Can you work these out from the model? Positions are in its coordinate system, mm. A direction names the side the tool comes from. Give positions to 0.01 mm unless a question says otherwise; leave off trailing zeros. Loops run counter-clockwise (first coordinate to the right, second up) from the corner with the lowest first, then second, coordinate; pieces in that order, holes last. Notation, with made-up numbers: (49.5, -28.5) - (91.5, -28.5) arc R25 cw to (91.5, -10.5) - close; hole circle Ø9 at (-37, 86). An arc over 180 degrees is marked (long way). Answer as a JSON object with one key per item and string values. Group by question number.
Item 1: Which directions (+Z, -Z, +X, -X, +Y, -Y) give clear straight access to the entire face, cutting with the end or side of a thin tool? Please do faces 5 (the cylindrical face through (-0.314, -14.284, 3.863)), 6 (the cylindrical face through (6.983, 43.545, 3.863)), 7 (the flat face through (-9, 51.243, 4)).
Item 2: Suppose I cut it at B-B on y = 52.07. Write out the boundary of the cut face in (x, z), and give its area (3 significant figures).
Item 3: Please list where these lines run through material, in increasing order: L1, parallel to X at y = 52.5, z = 7.25; L2, parallel to Y at x = -7, z = 2.5; L3, parallel to X at y = 17.5, z = 1.25.
Item 4: Suppose I cut it at C-C on z = 1.5. Count the separate pieces of the cut face and the enclosed holes in it, and give its area (3 significant figures).
Item 5: Thinking about a two-plate mould opening in X: for faces 1 (the cylindrical face through (-11.94, 52.05, 3.86)), 2 (the flat face through (-3, 44.45, 4)), 3 (the flat face through (14.288, 27, 4)), 4 (the cylindrical face through (0.175, -7.936, 3.863)), which applies, pulls with the +X half, pulls with the -X half, needs draft (parallel to the pull), parting line crosses it, or undercut?
Item 6: Suppose I cut it at D-D on y = 2. Write out the boundary of the cut face in (x, z).
Item 7: Will these pins go through, and if not, where does the flat tip stop? pin 1 (2.5 mm diameter, centred on x = -2.5, z = 2.5, fed in from -Y); pin 2 (2.5 mm diameter, centred on y = 11.5, z = 2.5, fed in from -X); pin 3 (4 mm diameter, centred on x = -8, z = 3.5, fed in from +Y).
from build123d import *

# Parameters (mm, degrees)
F1_DEPTH = 3.81
F2_R     = 22.225
F3_DEPTH = 109
F4_DEPTH = 28.576


# Not quite as in the source:
# - an extrude ends at something that could not be found from the text; its depth is read off the source's solid
# - a pattern or mirror of a feature is missing from the dataset's text; its kind, count and spacing are read off the source's solid


with BuildPart() as f1:
    # F0 (on Top) → F1 (new body)
    with BuildSketch(Plane.XY):
        with BuildLine():
            ThreePointArc((7.9375, 0), (0, -7.9375), (-7.9375, 0))
            ThreePointArc((-7.9375, 0), (-8.8674359697, 2.2450640303), (-11.1125, 3.175))
            ThreePointArc((-11.1125, 3.175), (-13.3575640303, 2.2450640303), (-14.2875, 0))
            ThreePointArc((-14.2875, 0), (0, -14.2875), (14.2875, 0))
            Line((14.2875, 0), (14.2875, 53.975))
            ThreePointArc((14.2875, 53.975), (13.3575640303, 56.2200640303), (11.1125, 57.15))
            Line((11.1125, 57.15), (-11.1125, 57.15))
            ThreePointArc((-11.1125, 57.15), (-13.3575640303, 56.2200640303), (-14.2875, 53.975))
            Line((-14.2875, 53.975), (-14.2875, 47.625))
            ThreePointArc((-14.2875, 47.625), (-13.3575640303, 45.3799359697), (-11.1125, 44.45))
            Line((-11.1125, 44.45), (4.7625, 44.45))
            ThreePointArc((4.7625, 44.45), (7.0075640303, 43.5200640303), (7.9375, 41.275))
            Line((7.9375, 41.275), (7.9375, 0))
        make_face()
        with BuildLine():
            ThreePointArc((-11.1125, 51.2426083993), (-11.9398916007, 52.07), (-11.1125, 52.8973916007))
            Line((-11.1125, 52.8973916007), (-6.3490160938, 52.8936081389))
            ThreePointArc((-6.3490160938, 52.8936081389), (-5.5241718233, 52.0677805671), (-6.3496717582, 51.2426083993))
            Line((-6.3496717582, 51.2426083993), (-11.1125, 51.2426083993))
        make_face(mode=Mode.SUBTRACT)
        with BuildLine():
            ThreePointArc((11.1133453348, 52.8905930346), (11.93309347, 52.07), (11.1133453348, 51.2494069654))
            Line((11.1133453348, 51.2494069654), (6.35, 51.2445))
            ThreePointArc((6.35, 51.2445), (5.5245, 52.07), (6.35, 52.8955))
            Line((6.35, 52.8955), (11.1133453348, 52.8905930346))
        make_face(mode=Mode.SUBTRACT)
    extrude(amount=F1_DEPTH)

    # F1_copies: F1 across plane


with BuildPart() as f1_1:
    add(f1.part)
    add(f1.part.mirror(Plane.XY.offset(3.81)))

    # F2 (on face) → F3 (cut, through all)
    with BuildSketch(Plane(origin=(-14.2875, 0, 0), x_dir=(0, -1, 0), z_dir=(-1, 0, 0))):
        with Locations((79.121, 3.81)):
            Circle(F2_R)
        with BuildLine():
            ThreePointArc((-57.15, 0.4595098866), (-56.9595909744, 2.1299479175), (-56.896, 3.81))
            ThreePointArc((-56.896, 3.81), (-101.2824090256, 5.4900520825), (-57.15, 0.4595098866))
        make_face()
    extrude(amount=F3_DEPTH, mode=Mode.SUBTRACT)

    # F2 (on face) → F4 (cut, through all)
    with BuildSketch(Plane(origin=(-14.2875, 0, 0), x_dir=(0, -1, 0), z_dir=(-1, 0, 0))):
        with Locations((79.121, 3.81)):
            Circle(F2_R)
        with BuildLine():
            ThreePointArc((-57.15, 0.4595098866), (-56.9595909744, 2.1299479175), (-56.896, 3.81))
            ThreePointArc((-56.896, 3.81), (-101.2824090256, 5.4900520825), (-57.15, 0.4595098866))
        make_face()
    extrude(amount=-F4_DEPTH, mode=Mode.SUBTRACT)


solid = f1_1.part
Worked out:
{
 "1": {"face 5": "+Z, -Z, -Y", "face 6": "+Z, -Z, -X", "face 7": "+Z, -Z"},
 "2": {"outline": "(-14.29, 0) - (-11.94, 0) - (-11.94, 7.62) - (-14.29, 7.62) - close; (-5.52, 0) - (5.52, 0) - (5.52, 7.62) - (-5.52, 7.62) - close; (11.93, 0) - (14.29, 0) - (14.29, 7.62) - (11.93, 7.62) - close", "area": "120 mm2"},
 "3": {"L1": "x = -14.29 to -11.82, -5.65 to 5.65, 11.81 to 14.29", "L2": "y = -12.46 to -3.74, 44.45 to 51.24, 52.89 to 56.93", "L3": "x = 7.94 to 14.29"},
 "4": {"separate pieces": "1", "enclosed holes": "2", "area": "855 mm2"},
 "5": {"face 1": "undercut", "face 2": "needs draft", "face 3": "pulls with the +X half", "face 4": "undercut"},
 "6": {"outline": "(-13.58, 0) - (-8.65, 0) - (-8.65, 7.62) - (-13.58, 7.62) - close; (7.94, 0) - (14.29, 0) - (14.29, 7.62) - (7.94, 7.62) - close"},
 "7": {"pin 1": "stops at y = -14.23", "pin 2": "stops at x = 7.94", "pin 3": "stops at y = 57.02"}
}
